```python
from build123d import *

# Parameters (mm, degrees)
SKETCH_1_W             = 160
SKETCH_1_H             = 210
SKETCH_1_R             = 11.5
SM_BASE_FLANGE_1_DEPTH = 16


# Sheet-metal steps are written as plain solids
with BuildPart() as part:
    # Sketch 1 → Базовая кромка1 (new body)
    with BuildSketch(Plane.XY):
        with Locations((80, -105)):
            Rectangle(SKETCH_1_W, SKETCH_1_H)
        with Locations((30, -55)):
            Circle(SKETCH_1_R, mode=Mode.SUBTRACT)
        with Locations(Location((130, -55, 0), (0, 0, 180))):
            Circle(SKETCH_1_R, mode=Mode.SUBTRACT)
        with Locations((130, -155)):
            Circle(SKETCH_1_R, mode=Mode.SUBTRACT)
        with Locations(Location((30, -155, 0), (0, 0, 180))):
            Circle(SKETCH_1_R, mode=Mode.SUBTRACT)
    extrude(amount=-SM_BASE_FLANGE_1_DEPTH)


solid = part.part
```
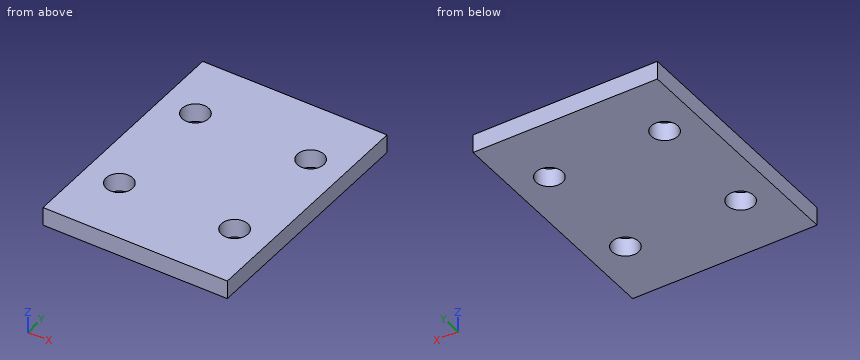
Work out the finished part from the listing and answer in its coordinate system (mm). Round coordinates to 2 decimals unless told otherwise and drop trailing zeros. Loops run counter-clockwise (first coordinate to the right, second up) from the corner with the lowest first, then second, coordinate; pieces in that order, holes last. Notation, with made-up numbers: (38.25, 51) -> (53.25, 51) arc R26 cw to (53.25, 87) -> close; hole circle Ø4 at (13.5, 88.25). An arc over 180 degrees is marked (long way). Write each question's results on one line, items separated by ' | '. Start each with the question number.
1. Given pin 1 Ø14 at (x, y) = (30, -155) entering from -Z, flat-ended and moving along its own axis, determine where the tip first touches the part or whether it passes through.
2. Section B-B (x = 130) is taken. Determine the outline of the cut face in (y, z).
3. Section A-A (y = -155) is taken. Determine the outline of the cut face in (x, z).
4. Section C-C (z = -8.25) is taken. Determine the outline of the cut face in (x, y).
5. Find the intervals of material crossed by probe 1 along Y at (x, z) = (30, -4.5); probe 2 along X at (y, z) = (-50, -2); probe 3 along X at (y, z) = (-153.5, -9), in increasing order. Write a range as from..to.
Evaluation:
1) pin 1: passes through
2) outline: (-210, -16) -> (-166.5, -16) -> (-166.5, 0) -> (-210, 0) -> close; (-143.5, -16) -> (-66.5, -16) -> (-66.5, 0) -> (-143.5, 0) -> close; (-43.5, -16) -> (0, -16) -> (0, 0) -> (-43.5, 0) -> close
3) outline: (0, -16) -> (18.5, -16) -> (18.5, 0) -> (0, 0) -> close; (41.5, -16) -> (118.5, -16) -> (118.5, 0) -> (41.5, 0) -> close; (141.5, -16) -> (160, -16) -> (160, 0) -> (141.5, 0) -> close
4) outline: (0, -210) -> (160, -210) -> (160, 0) -> (0, 0) -> close; hole circle Ø23 at (30, -155); hole circle Ø23 at (30, -55); hole circle Ø23 at (130, -155); hole circle Ø23 at (130, -55)
5) probe 1: y = -210..-166.5, -143.5..-66.5, -43.5..0 | probe 2: x = 0..19.64, 40.36..119.64, 140.36..160 | probe 3: x = 0..18.6, 41.4..118.6, 141.4..160
